Geometry: see drawing. Coordinates: mm, zero at the bounding-box minimum. Coordinates: 2 decimals unless noted, no trailing zeros. Write each loop counter-clockwise with the first axis right and the second up, starting at its lowest first coordinate (ties: lowest second). Pieces come first, ordered by that corner, then holes.
1) Pin query (flat end, axial travel): pin 1 Ø3 at (x, y) = (11.03, 72.5) entering from +Z; pin 2 Ø4 at (x, z) = (28, 4.5) entering from -Y; pin 3 Ø1 at (x, z) = (24.5, 22) entering from +Y; pin 4 Ø3.5 at (x, y) = (50, 5) entering from +Z. Return the tip coordinate at first contact, or that it passes through.
2) Section query A-A (y = 50). Output: boundary loops of the cut face in (x, z), then the cut area to 3 significant figures.
3) Draft query along Y for the marked faces 1, 2 and 3. Return one class per face: pulls with the +Y half, pulls with the -Y half, needs draft (parallel to the pull), parting line crosses it, or undercut.
4) Section query D-D (z = 7.5). Output: boundary loops of the cut face in (x, y).
5) Line query: L1, parallel to Y at x = 50, z = 0.6; L2, parallel to Y at x = 50, z = 17.5; L3, parallel to X at y = 72.5, z = 0.6. Output: solid intervals per line, ascending.
6) Section query B-B (x = 50). Output: boundary loops of the cut face in (y, z), then the cut area to 3 significant figures.
7) Section query C-C (x = 66). Output: boundary loops of the cut face in (y, z).
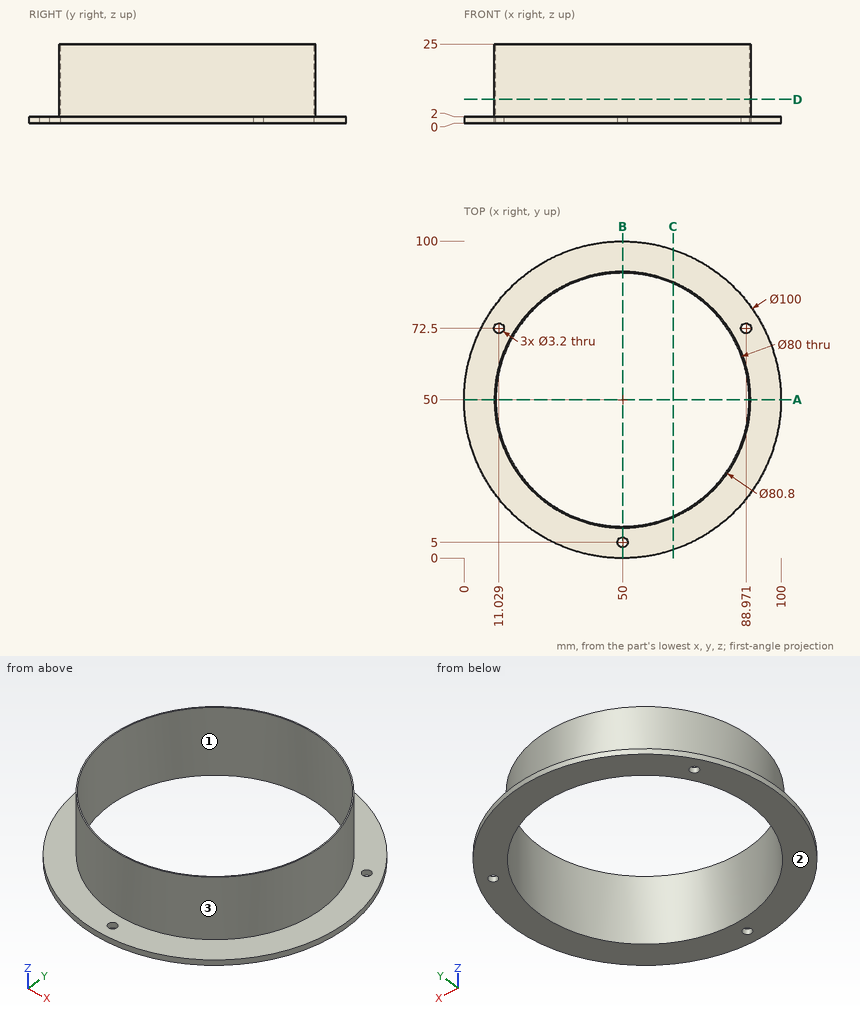
Answer:
1. pin 1: passes through
1. pin 2: stops at y = 14.9
1. pin 3: stops at y = 81.74
1. pin 4: stops at z = 2
2. outline: (0, 0) - (10, 0) - (10, 25) - (9.6, 25) - (9.6, 2) - (0, 2) - close; (90, 0) - (100, 0) - (100, 2) - (90.4, 2) - (90.4, 25) - (90, 25) - close
2. area: 58.4 mm2
3. face 1: undercut
3. face 2: needs draft
3. face 3: parting line crosses it
4. outline: circle Ø80.8 at (50, 50); hole circle Ø80 at (50, 50)
5. L1: y = 0 to 3.4, 6.6 to 10, 90 to 100
5. L2: y = 9.6 to 10, 90 to 90.4
5. L3: x = 5.35 to 9.43, 12.63 to 16.93, 83.07 to 87.37, 90.57 to 94.65
6. outline: (0, 0) - (3.4, 0) - (3.4, 2) - (0, 2) - close; (6.6, 0) - (10, 0) - (10, 25) - (9.6, 25) - (9.6, 2) - (6.6, 2) - close; (90, 0) - (100, 0) - (100, 2) - (90.4, 2) - (90.4, 25) - (90, 25) - close
6. area: 52.0 mm2
7. outline: (2.63, 0) - (13.34, 0) - (13.34, 25) - (12.9, 25) - (12.9, 2) - (2.63, 2) - close; (86.66, 0) - (97.37, 0) - (97.37, 2) - (87.1, 2) - (87.1, 25) - (86.66, 25) - close
